from build123d import *

# Parameters (mm, degrees)
SKETCH1_W           = 25
SKETCH1_H           = 45
BOSS_EXTRUDE1_DEPTH = 3
CUT_EXTRUDE1_DEPTH  = 1
SKETCH3_R           = 1.5
CUT_EXTRUDE2_DEPTH  = 4


with BuildPart() as part:
    # Sketch1 → Boss-Extrude1 (new body)
    with BuildSketch(Plane(origin=(0, 0, 0), x_dir=(1, 0, 0), z_dir=(0, 1, 0))):
        with Locations((12.5, 22.5)):
            Rectangle(SKETCH1_W, SKETCH1_H)
    extrude(amount=BOSS_EXTRUDE1_DEPTH)

    # Sketch2 → Cut-Extrude1 (cut)
    with BuildSketch(Plane(origin=(0, 3, 0), x_dir=(1, 0, 0), z_dir=(0, 1, 0))):
        with BuildLine():
            Line((4, 40), (21, 40))
            ThreePointArc((21, 40), (23.121320344, 39.121320344), (24, 37))
            Line((24, 37), (24, 27.390411508))
            ThreePointArc((24, 27.390411508), (23.725985305, 25.065500788), (22.918958029, 22.868002009))
            Line((22.918958029, 22.868002009), (20.581041971, 18.257235294))
            ThreePointArc((20.581041971, 18.257235294), (19.774014695, 16.059736514), (19.5, 13.734825794))
            Line((19.5, 13.734825794), (19.5, 0))
            Line((19.5, 0), (5.5, 0))
            Line((5.5, 0), (5.5, 13.734825794))
            ThreePointArc((5.5, 13.734825794), (5.225985305, 16.059736514), (4.418958029, 18.257235294))
            Line((4.418958029, 18.257235294), (2.081041971, 22.868002009))
            ThreePointArc((2.081041971, 22.868002009), (1.274014695, 25.065500788), (1, 27.390411508))
            Line((1, 27.390411508), (1, 37))
            ThreePointArc((1, 37), (1.878679656, 39.121320344), (4, 40))
        make_face()
    extrude(amount=-CUT_EXTRUDE1_DEPTH, mode=Mode.SUBTRACT)

    # Sketch3 → Cut-Extrude2 (cut, through all)
    with BuildSketch(Plane(origin=(0, 3, 0), x_dir=(1, 0, 0), z_dir=(0, 1, 0))):
        with Locations((21, 42)):
            Circle(SKETCH3_R)
        with Locations((4, 42)):
            Circle(SKETCH3_R)
        with Locations((3, 4)):
            Circle(SKETCH3_R)
        with Locations((22, 4)):
            Circle(SKETCH3_R)
    extrude(amount=-CUT_EXTRUDE2_DEPTH, mode=Mode.SUBTRACT)


solid = part.part
The model under review builds one solid part; all positions refer to its coordinate system, in mm. A direction names the side the tool comes from. Coordinates: 2 decimals unless noted, no trailing zeros. Write each loop counter-clockwise with the first axis right and the second up, starting at its lowest first coordinate (ties: lowest second). Pieces come first, ordered by that corner, then holes. Notation, with made-up numbers: (58.5, 4) -> (75.5, 4) arc R23 ccw to (75.5, 26) -> close; hole circle Ø9 at (72, -24). An arc over 180 degrees is marked (long way). Answer in a Markdown table with one row per item.
1. For faces 4 (the flat face through (21.766, 2.507, -20.595)), 5 (the cylindrical face through (20.675, 1.521, -40.536)), 6 (the flat face through (5.5, 2.5, -6.8)), list the 3-axis set-ups (+Z, -Z, +X, -X, +Y, -Y) from which the entire face can be reached by the end or side of a thin tool; tool diameter is ignored.
Answers below:
| item | result |
|---|---|
| face 4 | +Y |
| face 5 | +Y, -Y |
| face 6 | +Z, +Y |
2. We need section B-B, the plane y = 0.9. State the section outline as (x, z) points, and give its area (3 significant figures).
Answers below:
| item | result |
|---|---|
| outline | (0, -45) -> (25, -45) -> (25, 0) -> (0, 0) -> close; hole circle Ø3 at (3, -4); hole circle Ø3 at (4, -42); hole circle Ø3 at (21, -42); hole circle Ø3 at (22, -4) |
| area | 1,100 mm^2 |
3. We need section D-D, the plane x = 3. State the section outline as (y, z) points, and give its area (3 significant figures).
Answers below:
| item | result |
|---|---|
| outline | (0, -45) -> (3, -45) -> (3, -43.12) -> (0, -43.12) -> close; (0, -40.88) -> (3, -40.88) -> (3, -39.83) -> (2, -39.83) -> (2, -21.06) -> (3, -21.06) -> (3, -5.5) -> (0, -5.5) -> close; (0, -2.5) -> (3, -2.5) -> (3, 0) -> (0, 0) -> close |
| area | 101 mm^2 |
4. Draft analysis for pull direction X (two halves, no side actions). For faces 1 (the flat face through (19.5, 2.5, -7)), 2 (the cylindrical face through (1.282, 2.507, -25.034)), 3 (the flat face through (4, 3, -18)), state which applies: +X half, -X half, draft (parallel to the pull), parting line (faces both ways), or undercut.
Answers below:
| item | result |
|---|---|
| face 1 | undercut |
| face 2 | undercut |
| face 3 | draft |
5. We need section A-A, the plane z = -4. State the section outline as (x, y) points.
Answers below:
| item | result |
|---|---|
| outline | (0, 0) -> (1.5, 0) -> (1.5, 3) -> (0, 3) -> close; (4.5, 0) -> (20.5, 0) -> (20.5, 3) -> (19.5, 3) -> (19.5, 2) -> (5.5, 2) -> (5.5, 3) -> (4.5, 3) -> close; (23.5, 0) -> (25, 0) -> (25, 3) -> (23.5, 3) -> close |
6. Clearance check with flat-ended pins moving along their axes: pin 1 Ø1.1 at (y, z) = (2.5, -10) entering from -X; pin 2 Ø1.8 at (x, z) = (4, -42) entering from +Y; pin 3 Ø2 at (x, z) = (18.5, -30) entering from +Y. State where each tip first meets the part, or that it passes through.
Answers below:
| item | result |
|---|---|
| pin 1 | stops at x = 0 |
| pin 2 | passes through |
| pin 3 | stops at y = 2 |
7. We need section C-C, the plane z = -35. State the section outline as (x, y) points, and give its area (3 significant figures).
Answers below:
| item | result |
|---|---|
| outline | (0, 0) -> (25, 0) -> (25, 3) -> (24, 3) -> (24, 2) -> (1, 2) -> (1, 3) -> (0, 3) -> close |
| area | 52.0 mm^2 |
8. Wall thickness on probe 1 along X at (y, z) = (1.4, -41); probe 2 along Z at (x, y) = (22, 1); probe 3 along X at (y, z) = (2.55, -41.5): over which ranges is each line inside the solid? List them lowest first. Write a range as [from, to].
Answers below:
| item | result |
|---|---|
| probe 1 | x = [0, 2.88], [5.12, 19.88], [22.12, 25] |
| probe 2 | z = [-45, -43.12], [-40.88, -5.5], [-2.5, 0] |
| probe 3 | x = [0, 2.59], [5.41, 19.59], [22.41, 25] |
